Design review of the part built by this model. Coordinates are the model's own, in mm. A direction names the side the tool comes from. Round coordinates to 2 decimals unless told otherwise and drop trailing zeros. Loops run counter-clockwise (first coordinate to the right, second up) from the corner with the lowest first, then second, coordinate; pieces in that order, holes last. Notation, with made-up numbers: (-16, 22) - (36, 22) arc R28 ccw to (36, 51) - close; hole circle Ø3 at (62, 88.25). An arc over 180 degrees is marked (long way). One line per question, with ' | ' between items. Start each with the question number.
from build123d import *

# Parameters (mm, degrees)
SKETCH_1_W          = 10
SKETCH_1_H          = 30
EXTRUDE_1_DEPTH     = 3
SKETCH_2_R          = 2.5
CUT_EXTRUDE_1_DEPTH = 3
FILLET_2_R          = 2.5
FILLET_3_R          = 2.5
SKETCH_3_W          = 10
SKETCH_3_H          = 3.011531622
EXTRUDE_2_DEPTH     = 8
SKETCH_4_R          = 1.6
CUT_EXTRUDE_2_DEPTH = 7
CUT_EXTRUDE_3_DEPTH = 2
FILLET_4_R          = 1.5


with BuildPart() as part:
    # Эскиз1 → Бобышка-Вытянуть1 (new body)
    with BuildSketch(Plane.XY):
        Rectangle(SKETCH_1_W, SKETCH_1_H)
    extrude(amount=EXTRUDE_1_DEPTH)

    # Эскиз2 → Вырез-Вытянуть1 (cut)
    with BuildSketch(Plane(origin=(0, 0, 0), x_dir=(-1, 0, 0), z_dir=(0, 0, -1))):
        with Locations((0, 10)):
            Circle(SKETCH_2_R)
    extrude(amount=-CUT_EXTRUDE_1_DEPTH, mode=Mode.SUBTRACT)

    # Скругление2
    fillet_2_edges = [part.edges().sort_by_distance(p)[0] for p in [
        (5, 15, 1.5),
    ]]
    fillet(fillet_2_edges, radius=FILLET_2_R)

    # Скругление3
    fillet_3_edges = [part.edges().sort_by_distance(p)[0] for p in [
        (-5, 15, 1.5),
    ]]
    fillet(fillet_3_edges, radius=FILLET_3_R)

    # Эскиз3 → Бобышка-Вытянуть2 (add)
    with BuildSketch(Plane.XY.offset(3)):
        with Locations((0, -13.494234189)):
            Rectangle(SKETCH_3_W, SKETCH_3_H)
    extrude(amount=EXTRUDE_2_DEPTH)

    # Эскиз4 → Вырез-Вытянуть2 (cut)
    with BuildSketch(Plane(origin=(0, -11.988468378, 0), x_dir=(1, 0, 0), z_dir=(0, 1, 0))):
        with Locations(Location((0, -7.259187187, 0), (0, 0, 270))):
            Circle(SKETCH_4_R)
    extrude(amount=-CUT_EXTRUDE_2_DEPTH, mode=Mode.SUBTRACT)

    # Эскиз6 → Вырез-Вытянуть3 (cut)
    with BuildSketch(Plane(origin=(0, -11.988468378, 0), x_dir=(1, 0, 0), z_dir=(0, 1, 0))):
        Polygon((2.9, -8.933502968), (2.9, -5.584871406), (0, -3.910555626), (-2.9, -5.584871406), (-2.9, -8.933502968), (0, -10.607818748), align=None)
    extrude(amount=-CUT_EXTRUDE_3_DEPTH, mode=Mode.SUBTRACT)

    # Скругление4
    # the kernel refuses this fillet: 1.5 mm, written as the material it adds along each edge
    with BuildSketch(Plane(origin=(5, -11.988468378, 3), x_dir=(0, 1, 0), z_dir=(-1, 0, 0))) as fillet_4_piece_1_section:
        with BuildLine():
            CenterArc((FILLET_4_R, -FILLET_4_R), FILLET_4_R, 90, 90)
            Line((0, -FILLET_4_R), (0, 0))
            Line((0, 0), (FILLET_4_R, 0))
        make_face()
    fillet_4_piece_1 = extrude(amount=10, mode=Mode.PRIVATE)
    fillet_4_piece_1 = split(fillet_4_piece_1, bisect_by=Plane(origin=(2.478209897, -11.671443833, 2.479760474), z_dir=(0.49999999999999983, 0, 0.8660254037844388)), keep=Keep.TOP, mode=Mode.PRIVATE)
    fillet_4_piece_1 = split(fillet_4_piece_1, bisect_by=Plane(origin=(2.013101716, -11.671443833, 5.072820443), z_dir=(0.49999999999999994, 0, -0.8660254037844387)), keep=Keep.TOP, mode=Mode.PRIVATE)
    add(fillet_4_piece_1)
    with BuildSketch(Plane(origin=(5, -11.988468378, 3), x_dir=(0, 1, 0), z_dir=(-1, 0, 0))) as fillet_4_piece_2_section:
        with BuildLine():
            CenterArc((FILLET_4_R, -FILLET_4_R), FILLET_4_R, 90, 90)
            Line((0, -FILLET_4_R), (0, 0))
            Line((0, 0), (FILLET_4_R, 0))
        make_face()
    fillet_4_piece_2 = extrude(amount=10, mode=Mode.PRIVATE)
    fillet_4_piece_2 = split(fillet_4_piece_2, bisect_by=Plane(origin=(0.3145023, -11.552147507, 3.728977638), z_dir=(-0.49999999999999983, 0, -0.8660254037844388)), keep=Keep.TOP, mode=Mode.PRIVATE)
    fillet_4_piece_2 = split(fillet_4_piece_2, bisect_by=Plane(origin=(-0.3145023, -11.552147507, 3.728977638), z_dir=(0.49999999999999994, 0, -0.8660254037844387)), keep=Keep.TOP, mode=Mode.PRIVATE)
    add(fillet_4_piece_2)
    with BuildSketch(Plane(origin=(5, -11.988468378, 3), x_dir=(0, 1, 0), z_dir=(-1, 0, 0))) as fillet_4_piece_3_section:
        with BuildLine():
            CenterArc((FILLET_4_R, -FILLET_4_R), FILLET_4_R, 90, 90)
            Line((0, -FILLET_4_R), (0, 0))
            Line((0, 0), (FILLET_4_R, 0))
        make_face()
    fillet_4_piece_3 = extrude(amount=10, mode=Mode.PRIVATE)
    fillet_4_piece_3 = split(fillet_4_piece_3, bisect_by=Plane(origin=(-2.013101716, -11.671443833, 5.072820443), z_dir=(-0.49999999999999983, 0, -0.8660254037844388)), keep=Keep.TOP, mode=Mode.PRIVATE)
    fillet_4_piece_3 = split(fillet_4_piece_3, bisect_by=Plane(origin=(-2.478209897, -11.671443833, 2.479760474), z_dir=(-0.49999999999999994, 0, 0.8660254037844387)), keep=Keep.TOP, mode=Mode.PRIVATE)
    add(fillet_4_piece_3)


solid = part.part
1. Take a section at A-A, the plane y = 10. Give the boundary of the cut face in (x, z), then the cut area to 3 significant figures.
2. Take a section at D-D, the plane z = 8. Give the boundary of the cut face in (x, y).
3. Machinability: for faces 1 (the face through (0, 2, 3)), 2 (the face through (-1.47, -12.97, 9.76)), 3 (the face through (0.54, 7.56, 1.48)), which of the approach directions +Z, -Z, +X, -X, +Y, -Y give a long, thin tool a straight path to every point of the face, cutting with its end or side? Answer none if there is none.
4. Clearance check with flat-ended pins moving along their axes: P1, Ø1.5, axis at x = 1, z = 7, coming from the +Y side; P2, Ø3.5, axis at x = 0, z = 7.26, coming from the -Y side; P3, Ø3, axis at y = 1.5, z = 5.5, coming from the -X side; P4, Ø4.5, axis at x = 0.5, z = 8, coming from the +Y side. State where each tip first meets the part, or that it passes through.
5. Take a section at C-C, the plane z = 2. Give the boundary of the cut face in (x, y).
6. Take a section at B-B, the plane x = -0.75. Give the boundary of the cut face in (y, z).
7. To check wall thickness, follow line 1 along Y through (x, z) = (0, 0.7); line 2 along Z through (x, y) = (-3.75, -10.5); line 3 along Y through (x, z) = (-2, 7.75). State the ranges of each line that lie inside material, in increasing order.
8. The part is to be moulded in two halves that separate along X. For faces 4 (the face through (0.07, -14.49, 5.66)), 5 (the face through (-5, -4, 2)), 6 (the face through (4.248, 14.287, 1.521)), say which applies: pulls with the +X half, pulls with the -X half, needs draft (parallel to the pull), parting line crosses it, or undercut.
Answer list:
1) outline: (-5, 0) - (-2.5, 0) - (-2.5, 3) - (-5, 3) - close; (2.5, 0) - (5, 0) - (5, 3) - (2.5, 3) - close | area: 15.0 mm²
2) outline: (-5, -15) - (-1.42, -15) - (-1.42, -13.99) - (-2.9, -13.99) - (-2.9, -11.99) - (-5, -11.99) - close; (1.42, -15) - (5, -15) - (5, -11.99) - (2.9, -11.99) - (2.9, -13.99) - (1.42, -13.99) - close
3) face 1: +Z, +X, -X, +Y | face 2: +Y | face 3: +Z, -Z
4) P1: stops at y = -13.99 | P2: stops at y = -15 | P3: passes through | P4: stops at y = -11.99
5) outline: (-5, -15) - (5, -15) - (5, 12.5) arc R2.5 ccw to (2.5, 15) - (-2.5, 15) arc R2.5 ccw to (-5, 12.5) - close; hole circle Ø5 at (0, 10)
6) outline: (-15, 0) - (7.62, 0) - (7.62, 3) - (-10.49, 3) arc R1.5 cw to (-11.98, 4.34) - (-13.99, 4.34) - (-13.99, 5.85) - (-15, 5.85) - close; (-15, 8.67) - (-13.99, 8.67) - (-13.99, 10.17) - (-11.99, 10.17) - (-11.99, 11) - (-15, 11) - close; (12.38, 0) - (15, 0) - (15, 3) - (12.38, 3) - close
7) line 1: y = -15 to 7.5, 12.5 to 15 | line 2: z = 0 to 3 | line 3: y = -15 to -13.99
8) face 4: undercut | face 5: pulls with the -X half | face 6: pulls with the +X half
